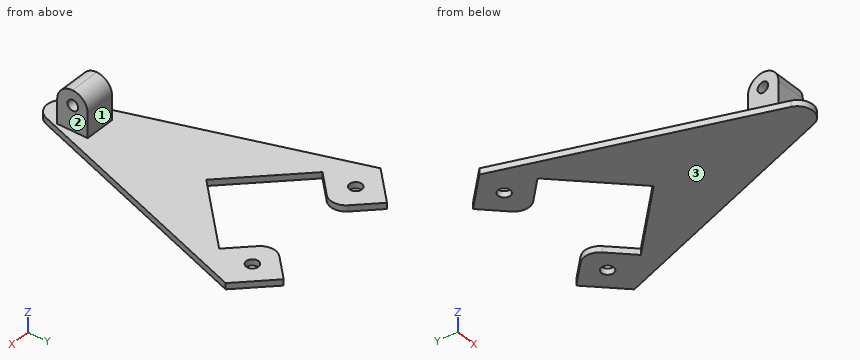
from build123d import *

# Parameters (mm, degrees)
F0_R     = 2
F1_DEPTH = 2
F2_ANGLE = 45
F3_W     = 10
F3_H     = 15
F3_R     = 1.75
F4_DEPTH = 5
F5_R     = 4.99999
F6_R     = 5


# Not quite as in the source:
# - a fillet or chamfer is up to 0.001 mm smaller than in the source, because OpenCascade refuses the exact size


with BuildPart() as f1:
    # F0 (on Top) → F1 (new body)
    with BuildSketch(Plane.XY):
        Polygon((0, 0), (-30, 0), (-30, 15), (-45, 15), (-45, 0), (44.535438389, -44.535438389), (0, 45), (-15, 45), (-15, 30), (0, 30), align=None)
        with Locations((-37.8073789179, 7.1926233359)):
            Circle(F0_R, mode=Mode.SUBTRACT)
        with Locations((-7.745902054, 37.5)):
            Circle(F0_R, mode=Mode.SUBTRACT)
    extrude(amount=F1_DEPTH)


with BuildPart() as f1_1:
    # F2: moved
    add(f1.part.rotate(Axis((0, 0, 1), (0, 0, -1)), F2_ANGLE))

    # F3 (on Right) → F4 (join, symmetric)
    with BuildSketch(Plane.YZ):
        with Locations((-40, 7.5)):
            Rectangle(F3_W, F3_H)
        with Locations((-39.8841314018, 10.2421231568)):
            Circle(F3_R, mode=Mode.SUBTRACT)
    extrude(amount=F4_DEPTH, both=True)

    # F5 (radius 5 in the source; OpenCascade refuses exactly that, so slightly less here)
    f5_edges = [f1_1.edges().sort_by_distance(p)[0] for p in [
        (0, -45, 15),
        (0, -35, 15),
        (10.606602, 31.819805, 1),
        (-10.606602, 31.819805, 1),
    ]]
    fillet(f5_edges, radius=F5_R)

    # F6
    f6_edges = [f1_1.edges().sort_by_distance(p)[0] for p in [
        (0, -62.982621, 1),
    ]]
    fillet(f6_edges, radius=F6_R)


solid = f1_1.part
Design review of the part built by this model. Coordinates are the model's own, in mm. Face numbers are marked on the shaded views. A direction names the side the tool comes from. Round coordinates to 2 decimals unless told otherwise and drop trailing zeros. Write each loop counter-clockwise with the first axis right and the second up, starting at its lowest first coordinate (ties: lowest second). Pieces come first, ordered by that corner, then holes. Notation, with made-up numbers: (83, -16) - (133, -16) arc R18 cw to (133, -4) - close; hole circle Ø9 at (66, -31). An arc over 180 degrees is marked (long way). Return JSON: item names as keys, results as strings. Group by question number.
Item 1: We need section D-D on y = 26. Write out the cut boundary in (x, z), and give its area (3 significant figures).
Item 2: We need section A-A on y = 15.5. Write out the cut boundary in (x, z), and give its area (3 significant figures).
Item 3: Insertion check: P1, Ø4.5, axis at y = -39.88, z = 10.24, coming from the -X side; P2, Ø3, axis at y = -39.5, z = 7.5, coming from the +X side; P3, Ø5, axis at y = 32.5, z = 5.5, coming from the -X side; P4, Ø8, axis at y = 1, z = 2.5, coming from the +X side. Each pin has a flat end and moves straight along its axis. Give the tip position at first contact, or say it passes through.
Item 4: We need section C-C on z = 7. Write out the cut boundary in (x, y).
Item 5: Machinability: for the marked faces 1, 2 and 3, which of the approach directions +Z, -Z, +X, -X, +Y, -Y give a long, thin tool a straight path to every point of the face, cutting with its end or side? Answer none if there is none.
Item 6: For probe 1 along Z at (x, y) = (21.5, 26); probe 2 along X at (y, z) = (-42, 10.5); probe 3 along Y at (x, z) = (-2.5, 11.5), list the stretches that pass through material, from the lowest coordinate up. Write a range as [from, to].
Model answer:
{
 "1": {"outline": "(-29.87, 0) - (-16.43, 0) - (-16.43, 2) - (-29.87, 2) - close; (16.43, 0) - (29.87, 0) - (29.87, 2) - (16.43, 2) - close", "area": "53.8 mm²"},
 "2": {"outline": "(-26.34, 0) - (-15.5, 0) - (-15.5, 2) - (-26.34, 2) - close; (15.5, 0) - (26.34, 0) - (26.34, 2) - (15.5, 2) - close", "area": "43.4 mm²"},
 "3": {"P1": "stops at x = -5", "P2": "stops at x = 5", "P3": "passes through", "P4": "stops at x = 22.81"},
 "4": {"outline": "(-5, -45) - (5, -45) - (5, -35) - (-5, -35) - close"},
 "5": {"face 1": "+Z, +X, -X, +Y", "face 2": "+Z, +X, +Y, -Y", "face 3": "-Z, +X, -X, +Y, -Y"},
 "6": {"probe 1": "z = [0, 2]", "probe 2": "x = [-5, 5]", "probe 3": "y = [-44.77, -41.1], [-38.67, -35.23]"}
}
